The model under review builds one solid part; all positions refer to its coordinate system, in mm. Coordinates: 2 decimals unless noted, no trailing zeros. Order: outer loops, then holes, each group sorted by start corner. A loop starts at its lowest first (then second) coordinate and runs counter-clockwise, first axis right, second up. Notation, with made-up numbers: (73.25, 59) -> (93.25, 59) arc R32 ccw to (93.25, 92) -> close; hole circle Ø6 at (12, 14). An arc over 180 degrees is marked (long way). Answer as CSV lines item,"result". Start each with the question number.
from build123d import *

# Parameters (mm, degrees)
SKETCH1_W           = 30
SKETCH1_H           = 120
BOSS_EXTRUDE1_DEPTH = 200
SKETCH2_OUTSIDE_W   = 79.032
SKETCH2_OUTSIDE_H   = 169.032
CUT_EXTRUDE2_DEPTH  = 210.344214155
FILLET1_R           = 5
CUT_EXTRUDE3_DEPTH  = 210.344214155
SKETCH4_R           = 2
CUT_EXTRUDE4_DEPTH  = 209.92343095


with BuildPart() as part:
    # Sketch1 → Boss-Extrude1 (new body)
    with BuildSketch(Plane(origin=(0, 0, 0), x_dir=(1, 0, 0), z_dir=(0, 1, 0))):
        Rectangle(SKETCH1_W, SKETCH1_H)
    extrude(amount=BOSS_EXTRUDE1_DEPTH)

    # Sketch2 outside → Cut-Extrude2 (cut, through all)
    with BuildSketch(Plane(origin=(0, 200, 0), x_dir=(1, 0, 0), z_dir=(0, 1, 0))):
        Rectangle(SKETCH2_OUTSIDE_W, SKETCH2_OUTSIDE_H)
        Polygon((0, 60), (-15, 34.019237886), (-15, -60), (15, -60), (15, 34.019237886), align=None, mode=Mode.SUBTRACT)
    extrude(amount=-CUT_EXTRUDE2_DEPTH, mode=Mode.SUBTRACT)

    # Fillet1
    fillet1_edges = [part.edges().sort_by_distance(p)[0] for p in [
        (0, 100, -60),
    ]]
    fillet(fillet1_edges, radius=FILLET1_R)

    # Sketch3 → Cut-Extrude3 (cut, through all)
    with BuildSketch(Plane(origin=(0, 200, 0), x_dir=(1, 0, 0), z_dir=(0, 1, 0))):
        Polygon((-15, 34.019237886), (-15, -60), (-7, -60), (-7, 47.875644347), align=None)
        Polygon((7, 47.875644347), (7, -60), (15, -60), (15, 34.019237886), align=None)
    extrude(amount=-CUT_EXTRUDE3_DEPTH, mode=Mode.SUBTRACT)

    # Sketch4 → Cut-Extrude4 (cut, through all)
    with BuildSketch(Plane.XZ):
        with Locations(Location((0, -46, 0), (0, 0, 270))):
            Circle(SKETCH4_R)
    extrude(amount=-CUT_EXTRUDE4_DEPTH, mode=Mode.SUBTRACT)


solid = part.part
1) Consider section A-A (x = 0). Give the boundary of the cut face in (y, z), plus the area to 3 significant figures.
2) Wall thickness on L1, parallel to X at y = 62, z = -46; L2, parallel to Z at x = -1.5, y = 136; L3, parallel to Z at x = -0.75, y = 66: over which ranges is each line inside the solid? List them lowest first. Write a range as [from, to].
3) Insertion check: pin 1 Ø3 at (x, z) = (0, -46) entering from +Y. The pin has a flat end and moves straight along its axis. Give the tip position at first contact, or say it passes through.
4) Consider section B-B (z = -46). Give the boundary of the cut face in (x, y).
5) Mouldability with a two-part tool opening along X and no side actions: class faces 1 (the face through (0, 99, 60)), 2 (the face through (5.68, 101.4, -50.16)), 3 (the face through (0, 99, -44)) as released by +X, released by -X, zero draft, split by the parting line, or undercut.
6) Consider section C-C (y = 75). Give the boundary of the cut face in (x, z), plus the area to 3 significant figures.
Result:
1,outline,"(0, -55) -> (200, -55) -> (200, -48) -> (0, -48) -> close; (0, -44) -> (200, -44) -> (200, 60) -> (0, 60) -> close"
1,area,"22,200 mm2"
2,L1,"[-7, -2], [2, 7]"
2,L2,"[-54.77, -47.32], [-44.68, 60]"
2,L3,"[-54.94, -47.85], [-44.15, 60]"
3,pin 1,"through"
4,outline,"(-7, 0) -> (-2, 0) -> (-2, 200) -> (-7, 200) -> close; (2, 0) -> (7, 0) -> (7, 200) -> (2, 200) -> close"
5,face 1,"zero draft"
5,face 2,"released by +X"
5,face 3,"undercut"
6,outline,"(-7, -47.88) -> (-4.33, -52.5) arc R5 ccw to (4.33, -52.5) -> (7, -47.88) -> (7, 60) -> (-7, 60) -> close; hole circle Ø4 at (0, -46)"
6,area,"1,570 mm2"
